from build123d import *

# Parameters (mm, degrees)
SKETCH1_R                = 57.15
BOSS_EXTRUDE3_DEPTH      = 2.54
CUT_EXTRUDE1_DEPTH       = 81.98179672
FILLET1_R                = 3.81
CIRPATTERN1_COUNT        = 6
FILLET1_OF_CIRPATTERN1_R = 3.81
CUT_EXTRUDE2_DEPTH       = 81.98179672
CUT_EXTRUDE2_DEPTH_BACK  = 81.98179672
SKETCH4_R                = 2.5
CUT_EXTRUDE3_DEPTH       = 2.667
SKETCH5_3_R              = 9
BOSS_EXTRUDE9_DEPTH      = 2.5
SKETCH11_R               = 2
CUT_EXTRUDE4_DEPTH       = 81.98179672


with BuildPart() as part:
    # Sketch1 → Boss-Extrude3 (new, symmetric)
    with BuildSketch(Plane.XY):
        Circle(SKETCH1_R)
    extrude(amount=BOSS_EXTRUDE3_DEPTH, both=True)

    # Sketch3 → Cut-Extrude1 (cut, symmetric)
    with BuildSketch(Plane.XY.offset(2.54)):
        with BuildLine():
            ThreePointArc((0, 11.43), (-5.277786649, 10.138533823), (-9.362907866, 6.555978667))
            Line((-9.362907866, 6.555978667), (-42.653246946, 29.866125041))
            ThreePointArc((-42.653246946, 29.866125041), (-28.641923541, 43.48476878), (-10.597439882, 50.980184071))
            Line((-10.597439882, 50.980184071), (0, 11.43))
        make_face()
    cut_extrude1 = extrude(amount=CUT_EXTRUDE1_DEPTH, both=True, mode=Mode.SUBTRACT)

    # Fillet1
    fillet1_edges = [part.edges().sort_by_distance(p)[0] for p in [
        (0, 11.43, 0),
        (-9.362907866, 6.555978667, 0),
        (-42.653246946, 29.866125041, 0),
        (-10.597439882, 50.980184071, 0),
    ]]
    fillet(fillet1_edges, radius=FILLET1_R)

    # CirPattern1: Cut-Extrude1 ×6 about axis
    cirpattern1_axis = Axis((0, 0, 0), (0, 0, 1))
    for i in range(1, CIRPATTERN1_COUNT):
        add(cut_extrude1.rotate(cirpattern1_axis, i * 360 / CIRPATTERN1_COUNT), mode=Mode.SUBTRACT)

    # Fillet1 of CirPattern1
    fillet1_of_cirpattern1_edges = [part.edges().sort_by_distance(p)[0] for p in [
        (-9.898670365, 5.715, 0),
        (-10.359098006, -4.830526732, 0),
        (-47.191446471, -22.005732889, 0),
        (-49.448854437, 16.312439882, 0),
        (-9.898670365, -5.715, 0),
        (-0.99619014, -11.386505399, 0),
        (-4.538199525, -51.87185793, 0),
        (-38.851414554, -34.667744189, 0),
        (0, -11.43, 0),
        (9.362907866, -6.555978667, 0),
        (42.653246946, -29.866125041, 0),
        (10.597439882, -50.980184071, 0),
        (9.898670365, -5.715, 0),
        (10.359098006, 4.830526732, 0),
        (47.191446471, 22.005732889, 0),
        (49.448854437, -16.312439882, 0),
        (9.898670365, 5.715, 0),
        (0.99619014, 11.386505399, 0),
        (4.538199525, 51.87185793, 0),
        (38.851414554, 34.667744189, 0),
    ]]
    fillet(fillet1_of_cirpattern1_edges, radius=FILLET1_OF_CIRPATTERN1_R)

    # Sketch4 → Cut-Extrude2 (cut, two sides: drawn at the far end of the back side and taken through both)
    with BuildSketch(Plane.XY.offset(2.54).offset(-CUT_EXTRUDE2_DEPTH_BACK)):
        Circle(SKETCH4_R)
    extrude(amount=CUT_EXTRUDE2_DEPTH + CUT_EXTRUDE2_DEPTH_BACK, mode=Mode.SUBTRACT)

    # Sketch5 → Cut-Extrude3 (cut, symmetric)
    with BuildSketch(Plane.XY.offset(2.54)):
        Polygon((4.515050808, -5.41450055), (6.946620429, 1.202898424), (2.431569621, 6.617398974), (-4.515050808, 5.41450055), (-6.946620429, -1.202898424), (-2.431569621, -6.617398974), align=None)
    extrude(amount=CUT_EXTRUDE3_DEPTH, both=True, mode=Mode.SUBTRACT)

    # Sketch5_3 → Boss-Extrude9 (add)
    with BuildSketch(Plane.XY.offset(2.54)):
        Circle(SKETCH5_3_R)
        Polygon((4.515050808, -5.41450055), (6.946620429, 1.202898424), (2.431569621, 6.617398974), (-4.515050808, 5.41450055), (-6.946620429, -1.202898424), (-2.431569621, -6.617398974), align=None, mode=Mode.SUBTRACT)
    extrude(amount=BOSS_EXTRUDE9_DEPTH)

    # Sketch11 → Cut-Revolve1 (revolve, cut)
    with BuildSketch(Plane(origin=(0, 0, 0), x_dir=(0, 0, -1), z_dir=(1, 0, 0)), mode=Mode.PRIVATE) as cut_revolve1_sk:
        with Locations((0, 57.15)):
            Circle(SKETCH11_R)
    revolve(cut_revolve1_sk.sketch.rotate(Axis((0, 0, 5.04), (0, 0, -1)), 90), axis=Axis((0, 0, 5.04), (0, 0, -1)), mode=Mode.SUBTRACT)

    # Sketch12 → Cut-Extrude4 (cut, through all)
    with BuildSketch(Plane.XY.offset(2.54)):
        Polygon((-48.637599982, 23.067154966), (-48.34382995, 23.643477082), (-45.821193732, 23.258561216), (-47.609054309, 25.08428237), (-47.319491007, 25.652191024), (-43.959715366, 24.596301601), (-44.249278668, 24.028392947), (-46.372976584, 24.692355287), (-44.75408636, 23.037707851), (-45.019110398, 22.518176601), (-47.30476745, 22.864530768), (-45.523216969, 21.52959487), (-45.815584757, 20.95537612), align=None)
        Polygon((47.301176757, -25.475850915), (47.59425656, -24.899177488), (45.798508906, -23.086129205), (48.326749768, -23.45721049), (48.615502847, -22.888889451), (45.784622613, -20.793868703), (45.495869534, -21.362189742), (47.282457589, -22.688478531), (44.991967867, -22.353335985), (44.727887152, -22.873347367), (46.352998071, -24.517489655), (44.225273466, -23.862688943), (43.933069043, -24.436990843), align=None)
    extrude(amount=-CUT_EXTRUDE4_DEPTH, mode=Mode.SUBTRACT)


solid = part.part
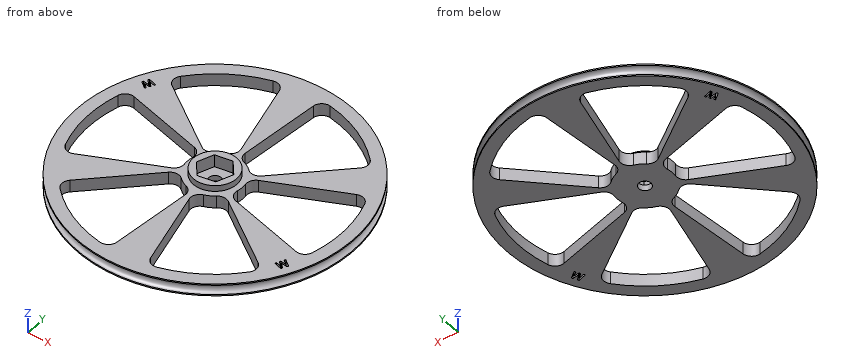
The listing builds one solid part. Answer for the finished solid, in the listing's coordinates (mm). Round coordinates to 2 decimals unless told otherwise and drop trailing zeros. Use a Markdown table: item, result. Add a question column.
1. Consider line 1 (Z direction, x = -24, y = 51.5); line 2 (Y direction, x = -33, z = 0.75); line 3 (Z direction, x = -43, y = 22.5). Determine where each line is inside the solid, lowest interval first.
2. Flat-ended cylindrical pins translate along their axes: P1, Ø4, axis at y = 7, z = -1, coming from the -X side; P2, Ø4, axis at x = 10.5, z = 0.5, coming from the +Y side; P3, Ø4, axis at x = -2.5, z = 2, coming from the +Y side. Find the tip coordinate at first contact, or state that the pin passes through.
3. The part is cut by section A-A (x = -28). Give the number of separate pieces and of enclosed holes in the cut face, and give its area (3 significant figures).
Reported:
| question | item | result |
|---|---|---|
| 1 | line 1 | -2.54 to -1.97, 1.97 to 2.54 |
| 1 | line 2 | -44.37 to -40.28, -28.82 to -15.39, 11.9 to 23.11, 40.28 to 44.37 |
| 1 | line 3 | -2.54 to 2.54 |
| 2 | P1 | x = -56.91 |
| 2 | P2 | y = 56.41 |
| 2 | P3 | y = 57.15 |
| 3 | separate pieces | 4 |
| 3 | enclosed holes | 0 |
| 3 | area | 146 mm^2 |
